```python
from build123d import *

# Parameters (mm, degrees)
SKETCH033_R     = 1.75
SKETCH033_R_2   = 3.7
PAD001_DEPTH    = 3
CHAMFER001_SIZE = 2
CHAMFER002_SIZE = 1.4


with BuildPart() as part:
    # Sketch033 → Pad001 (new body)
    with BuildSketch(Plane(origin=(0, -38, 0), x_dir=(1, 0, 0), z_dir=(0, -0.939693, 0.34202))):
        with BuildLine():
            Line((-34.406356, 37.6), (34.406361, 37.6))
            ThreePointArc((42.400003, 29.918894), (39.949322, 35.368499), (34.406361, 37.6))
            Line((42.400003, 29.918894), (43.15, 11.118894))
            ThreePointArc((35.156359, 2.8), (40.924857, 5.257038), (43.15, 11.118894))
            Line((35.156359, 2.8), (-35.156359, 2.8))
            ThreePointArc((-43.15, 11.118896), (-40.924858, 5.257039), (-35.156359, 2.8))
            Line((-43.15, 11.118896), (-42.399997, 29.918896))
            ThreePointArc((-34.406356, 37.6), (-39.949317, 35.368499), (-42.399997, 29.918896))
        make_face()
        with Locations((-36.75, 32.3)):
            Circle(SKETCH033_R, mode=Mode.SUBTRACT)
        with Locations((36.75, 32.3)):
            Circle(SKETCH033_R, mode=Mode.SUBTRACT)
        with Locations((-38, 8.3)):
            Circle(SKETCH033_R, mode=Mode.SUBTRACT)
        with Locations((38, 8.3)):
            Circle(SKETCH033_R, mode=Mode.SUBTRACT)
        with Locations((25, 22.9)):
            Circle(SKETCH033_R_2, mode=Mode.SUBTRACT)
        with BuildLine():
            Line((-11.75, 28.5), (7.75, 28.5))
            ThreePointArc((10, 26.25), (9.34099, 27.84099), (7.75, 28.5))
            Line((10, 26.25), (10, 17.65))
            ThreePointArc((7.75, 15.4), (9.34099, 16.05901), (10, 17.65))
            Line((7.75, 15.4), (-11.75, 15.4))
            ThreePointArc((-14, 17.65), (-13.34099, 16.05901), (-11.75, 15.4))
            Line((-14, 17.65), (-14, 26.25))
            ThreePointArc((-11.75, 28.5), (-13.34099, 27.84099), (-14, 26.25))
        make_face(mode=Mode.SUBTRACT)
        with BuildLine():
            Line((-29.35, 25.939165), (-24.65, 25.939165))
            ThreePointArc((-24.65, 14.680835), (-20.9, 20.31), (-24.65, 25.939165))
            Line((-29.35, 14.680835), (-24.65, 14.680835))
            ThreePointArc((-29.35, 25.939165), (-33.1, 20.31), (-29.35, 14.680835))
        make_face(mode=Mode.SUBTRACT)
    extrude(amount=PAD001_DEPTH)

    # Chamfer001
    chamfer001_edges = [part.edges().sort_by_distance(p)[0] for p in [
        (-2, -31.071504, 27.8073),
    ]]
    chamfer(chamfer001_edges, length=CHAMFER001_SIZE)

    # Chamfer002
    chamfer002_edges = [part.edges().sort_by_distance(p)[0] for p in [
        (-38.5, -29.771827, 31.378132),
        (-39.75, -37.980311, 8.825509),
        (35, -29.771827, 31.378132),
        (36.25, -37.980311, 8.825509),
    ]]
    chamfer(chamfer002_edges, length=CHAMFER002_SIZE)


solid = part.part
```
The listing builds one solid part. Answer for the finished solid, in the listing's coordinates (mm). A direction names the side the tool comes from. Coordinates: 2 decimals unless noted, no trailing zeros. Loops run counter-clockwise (first coordinate to the right, second up) from the corner with the lowest first, then second, coordinate; pieces in that order, holes last. Notation, with made-up numbers: (63, 30) -> (84, 30) arc R12 ccw to (84, 45) -> close; hole circle Ø5 at (52.25, -26). An arc over 180 degrees is marked (long way). Return JSON: item names as keys, results as strings. Group by question number.
(1) A cutting plane is placed at D-D on x = -31.5. Write down the section's boundary in (y, z).
(2) Find the intervals of material crossed by probe 1 along X at (y, z) = (-31.75, 19.5); probe 2 along X at (y, z) = (-31.5, 26); probe 3 along Y at (x, z) = (4, 4.5), in increasing order. Write a range as from..to.
(3) A cutting plane is placed at C-C on z = 19. Count the separate pieces of the cut face and the enclosed holes in it, and give its area (3 significant figures).
(4) A cutting plane is placed at A-A on x = -4.5. Write down the section's boundary in (y, z), and give its area (3 significant figures).
(5) A cutting plane is placed at B-B on x = 31. Write down the section's boundary in (y, z).
(6) Which of the six approach directions +Z, -Z, +X, -X, +Y, -Y give full straight-line access (tool end or side, diameter ignored) to faces 5 (the cylindrical face through (9.358, -28.947, 26.314)), 6 (the conical face through (9.877, -29.962, 27.323)), 7 (the conical face through (9.92, -34.37, 15.2)), 8 (the cylindrical face through (-13.358, -32.965, 15.276))?
(7) Determine the mould class of faces 1 (the flat face through (0.492, -38.432, 3.137)), 2 (the cylindrical face through (-33.1, -32.4, 19.7)), 3 (the cylindrical face through (40.011, -27.314, 33.685)), 4 (the cylindrical face through (-36.383, -36.132, 7.439)) for opening direction Z: released by +Z, released by -Z, zero draft, split by the parting line, or undercut.
(8) Given pin 1 Ø2 at (x, z) = (-20.5, 14) entering from +Y; pin 2 Ø1.2 at (y, z) = (-30.5, 20.5) entering from -X; pin 3 Ø8 at (x, z) = (-23, 9) entering from -Y, each flat-ended and moving along its own axis, determine where each tip first touches the part or whether it passes through.
The answers:
{
 "1": {"outline": "(-39.86, 3.66) -> (-37.04, 2.63) -> (-32.46, 15.22) -> (-35.28, 16.24) -> close; (-32.46, 23.98) -> (-29.65, 22.96) -> (-25.14, 35.33) -> (-27.96, 36.36) -> close"},
 "2": {"probe 1": "x = -42.78..-33.1, -20.9..-14, 10..22.22, 27.78..42.78", "probe 2": "x = -42.53..-15.76, 11.76..42.53", "probe 3": "y = -39.55..-36.36"},
 "3": {"separate pieces": "3", "enclosed holes": "0", "area": "143 mm^2"},
 "4": {"outline": "(-39.86, 3.66) -> (-37.04, 2.63) -> (-32.73, 14.47) -> (-33.67, 14.81) -> (-36.24, 13.62) -> close; (-30.39, 29.69) -> (-29.19, 27.12) -> (-28.25, 26.78) -> (-25.14, 35.33) -> (-27.96, 36.36) -> close", "area": "61.1 mm^2"},
 "5": {"outline": "(-39.86, 3.66) -> (-37.04, 2.63) -> (-25.14, 35.33) -> (-27.96, 36.36) -> close"},
 "6": {"face 5": "-Z, -Y", "face 6": "-Y", "face 7": "+Z, -Y", "face 8": "+Z, +Y"},
 "7": {"face 1": "released by -Z", "face 2": "undercut", "face 3": "released by +Z", "face 4": "undercut"},
 "8": {"pin 1": "stops at y = -32.54", "pin 2": "stops at x = -42.75", "pin 3": "stops at y = -39.37"}
}
